from build123d import *

# Parameters (mm, degrees)
SKETCH1_W           = 6.35
SKETCH1_H           = 50.8
BOSS_EXTRUDE1_START = 3.175
SKETCH2_R           = 57.15
BOSS_EXTRUDE1_DEPTH = 3.175


with BuildPart() as part:
    # Sketch1 → Revolve1 (revolve)
    with BuildSketch(Plane.XY, mode=Mode.PRIVATE) as revolve1_sk:
        with Locations((3.175, 25.4)):
            Rectangle(SKETCH1_W, SKETCH1_H)
    revolve(revolve1_sk.sketch.rotate(Axis((-50.8, 50.8, 0), (0, -1, 0)), 180), axis=Axis((-50.8, 50.8, 0), (0, -1, 0)))

    # Sketch2 → Boss-Extrude1 (add)
    with BuildSketch(Plane(origin=(0, 0, 0), x_dir=(1, 0, 0), z_dir=(0, 1, 0)).offset(BOSS_EXTRUDE1_START)):
        with Locations(Location((-50.8, 0, 0), (0, 0, 180))):
            Circle(SKETCH2_R)
    extrude(amount=-BOSS_EXTRUDE1_DEPTH)

    # Sketch4 → Cut-Revolve1 (revolve, cut)
    with BuildSketch(Plane.XY):
        with BuildLine():
            Line((-107.95, 50.8), (-50.8, 50.8))
            Line((-50.8, 50.8), (-50.8, 39.678581179))
            ThreePointArc((-50.8, 39.678581179), (-79.911030798, 42.484771528), (-107.95, 50.8))
        make_face()
    revolve(axis=Axis((-50.8, 46.230510517, 0), (0, 1, 0)), mode=Mode.SUBTRACT)


solid = part.part
CAD build for the part. Positions are in the model's coordinates, mm. Give positions to 0.01 mm unless a question says otherwise; leave off trailing zeros. Write each loop counter-clockwise with the first axis right and the second up, starting at its lowest first coordinate (ties: lowest second). Pieces come first, ordered by that corner, then holes. Notation, with made-up numbers: (-7, 20.5) -> (21, 20.5) arc R13 cw to (21, 40.5) -> close; hole circle Ø2 at (-14.75, -37.5). An arc over 180 degrees is marked (long way). Return JSON: item names as keys, results as strings.
Item 1: Band-saw the part on C-C (x = -19). List the corners of the cut face in (y, z) (3 decimals), then the cut area to 3 significant figures.
Answer below:
{"outline": "(0, -47.486) -> (50.8, -47.486) arc R149.045 cw to (48.394, -39.616) -> (3.175, -39.616) -> (3.175, 39.616) -> (48.394, 39.616) arc R149.045 cw to (50.8, 47.486) -> (0, 47.486) -> close", "area": "1,030 mm2"}
Item 2: Drill centre lines: probe 1 along Z at (x, y) = (-50.8, 34); probe 2 along Y at (x, z) = (-22, 26) (3 decimals); probe 3 along Z at (x, y) = (-48, 40.5). Where is each one in solid material? Low to high.
Answer below:
{"probe 1": "z = -57.15 to -50.8, 50.8 to 57.15", "probe 2": "y = 0 to 3.175", "probe 3": "z = -57.08 to -50.72, 50.72 to 57.08"}
Item 3: Band-saw the part on A-A (z = 0). List the corners of the cut face in (x, y) (3 decimals).
Answer below:
{"outline": "(-107.95, 0) -> (6.35, 0) -> (6.35, 50.8) arc R152.4 cw to (0, 48.394) -> (0, 3.175) -> (-101.6, 3.175) -> (-101.6, 48.394) arc R152.4 cw to (-107.95, 50.8) -> close"}
Item 4: Two-plate mould, pull along Z, no slides. Class faces 1 (the cylindrical face through (6.295, 25.756, -2.513)), 2 (the cylindrical face through (-74.24, 26.1, 45.07)), 3 (the flat face through (-52, 0, -1)): +Z half, -Z half, draft (parallel to the pull), parting line (faces both ways), or undercut.
Answer below:
{"face 1": "parting line", "face 2": "undercut", "face 3": "draft"}
Item 5: Band-saw the part on B-B (y = 12.5). List the corners of the cut face in (x, z).
Answer below:
{"outline": "circle Ø114.3 at (-50.8, 0); hole circle Ø101.6 at (-50.8, 0)"}
Item 6: Drop flat-ended pins along their axis: pin 1 (2 mm diameter, centred on y = 23, z = -9.5, fed in from -X); pin 2 (12 mm diameter, centred on x = -89.5, y = 21, fed in from +Z); pin 3 (4 mm diameter, centred on x = -77, z = -31.5, fed in from +Y) (3 decimals). Give the stop position or say it passes through.
Answer below:
{"pin 1": "stops at x = -107.31", "pin 2": "stops at z = 46.87", "pin 3": "stops at y = 3.175"}
